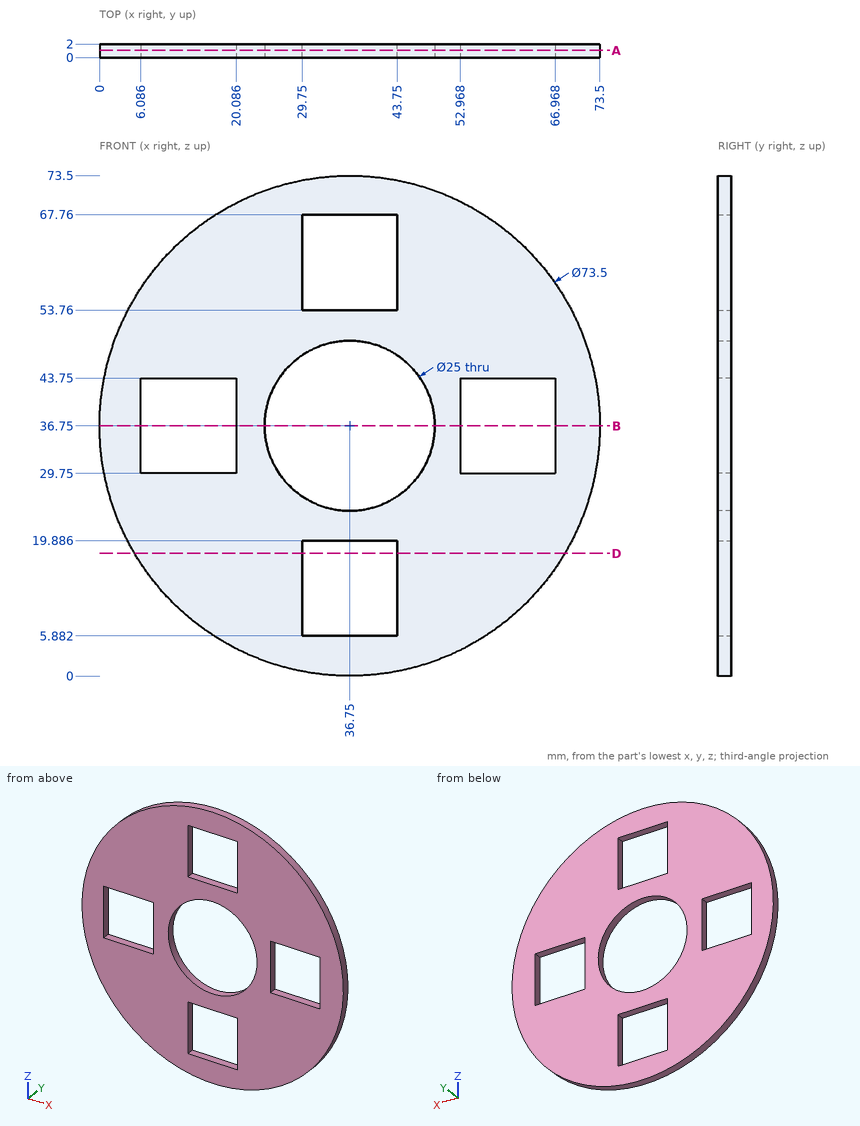
Input: dimensioned drawing with shaded views. Units: mm. Origin: part minimum x, y, z. Give positions to 0.01 mm unless a question says otherwise; leave off trailing zeros. Order: outer loops, then holes, each group sorted by start corner. A loop starts at its lowest first (then second) coordinate and runs counter-clockwise, first axis right, second up. Notation, with made-up numbers: (12.25, 63.25) -> (42.25, 63.25) arc R24 cw to (42.25, 94.25) -> close; hole circle Ø6 at (58.5, -28). An arc over 180 degrees is marked (long way). Answer as a JSON object with one key per item and string values.
Q1. Section D-D (z = 18). Output: boundary loops of the cut face in (x, y).
Entries:
{"outline": "(5.14, 0) -> (29.75, 0) -> (29.75, 2) -> (5.14, 2) -> close; (43.75, 0) -> (68.36, 0) -> (68.36, 2) -> (43.75, 2) -> close"}
Q2. Section B-B (z = 36.75). Output: boundary loops of the cut face in (x, y), plus the area to 3 significant figures.
Entries:
{"outline": "(0, 0) -> (6.09, 0) -> (6.09, 2) -> (0, 2) -> close; (20.09, 0) -> (24.25, 0) -> (24.25, 2) -> (20.09, 2) -> close; (49.25, 0) -> (52.97, 0) -> (52.97, 2) -> (49.25, 2) -> close; (66.97, 0) -> (73.5, 0) -> (73.5, 2) -> (66.97, 2) -> close", "area": "41.0 mm^2"}
Q3. Section A-A (y = 1.05). State how many separate pieces and enclosed holes the cut face has, plus the area to 3 significant figures.
Entries:
{"separate pieces": "1", "enclosed holes": "5", "area": "2,970 mm^2"}
Q4. First-contact query: pin 1 (5 mm diameter, centred on x = 10, z = 65, fed in from +Y); pin 2 (0.6 mm diameter, centred on x = 39.5, y = 1.5, fed in from -Z); pin 3 (1 mm diameter, centred on x = 16.5, y = 1.5, fed in from +Z); pin 4 (1 mm diameter, centred on x = 40, y = 1, fed in from +Z). Flat tips, straight axial feed; report the tip coordinate or a pass-through.
Entries:
{"pin 1": "stops at y = 2", "pin 2": "stops at z = 0.08", "pin 3": "stops at z = 67.74", "pin 4": "stops at z = 73.4"}
Q5. Material intervals for probe 1 along X at (y, z) = (0.5, 36.75); probe 2 along Z at (x, y) = (38, 1.35) (1 decimal); probe 3 along X at (y, z) = (1.75, 18.5), sorted ascending.
Entries:
{"probe 1": "x = 0 to 6.09, 20.09 to 24.25, 49.25 to 52.97, 66.97 to 73.5", "probe 2": "z = 0 to 5.9, 19.9 to 24.3, 49.2 to 53.8, 67.8 to 73.5", "probe 3": "x = 4.85 to 29.75, 43.75 to 68.65"}
